from build123d import *

# Parameters (mm, degrees)
SKETCH1_W           = 127
SKETCH1_H           = 101.6
BOSS_EXTRUDE1_DEPTH = 2.54
SKETCH2_W           = 76.2
SKETCH2_H           = 88.9
SKETCH2_W_2         = 34.29
SKETCH2_H_2         = 40.64
BOSS_EXTRUDE2_DEPTH = 6.35
SKETCH3_R           = 2.54
CUT_EXTRUDE1_DEPTH  = 163.763271348
CUT_EXTRUDE2_REACH  = 159.981
SKETCH4_W           = 42.672
SKETCH4_H           = 1.267041817
FILLET1_R           = 3.81
FILLET2_R           = 12.7
SKETCH5_R           = 0.635
CUT_EXTRUDE3_DEPTH  = 163.763271348


with BuildPart() as part:
    # Sketch1 → Boss-Extrude1 (new body)
    with BuildSketch(Plane(origin=(0, 0, 0), x_dir=(1, 0, 0), z_dir=(0, 1, 0))):
        with Locations((63.5, 50.8)):
            Rectangle(SKETCH1_W, SKETCH1_H)
    extrude(amount=BOSS_EXTRUDE1_DEPTH)

    # Sketch2 → Boss-Extrude2 (add)
    with BuildSketch(Plane(origin=(0, 2.54, 0), x_dir=(1, 0, 0), z_dir=(0, 1, 0))):
        with Locations((82.55, 50.8)):
            Rectangle(SKETCH2_W, SKETCH2_H)
        with Locations((64.135, 72.39)):
            Rectangle(SKETCH2_W_2, SKETCH2_H_2, mode=Mode.SUBTRACT)
        with Locations((64.135, 29.21)):
            Rectangle(SKETCH2_W_2, SKETCH2_H_2, mode=Mode.SUBTRACT)
        with Locations((100.965, 29.21)):
            Rectangle(SKETCH2_W_2, SKETCH2_H_2, mode=Mode.SUBTRACT)
        with Locations((100.965, 72.39)):
            Rectangle(SKETCH2_W_2, SKETCH2_H_2, mode=Mode.SUBTRACT)
    extrude(amount=BOSS_EXTRUDE2_DEPTH)

    # Sketch3 → Cut-Extrude1 (cut, through all)
    with BuildSketch(Plane(origin=(0, 2.54, 0), x_dir=(1, 0, 0), z_dir=(0, 1, 0))):
        with Locations(Location((64.135, 72.39, 0), (0, 0, 270))):
            Circle(SKETCH3_R)
        with Locations(Location((100.965, 72.39, 0), (0, 0, 270))):
            Circle(SKETCH3_R)
        with Locations(Location((64.135, 29.21, 0), (0, 0, 270))):
            Circle(SKETCH3_R)
        with Locations(Location((100.965, 29.21, 0), (0, 0, 270))):
            Circle(SKETCH3_R)
    extrude(amount=-CUT_EXTRUDE1_DEPTH, mode=Mode.SUBTRACT)

    # Cut-Extrude2: up to this face of the body (flat: up to its plane)
    cut_extrude2_end = Plane(part.part.faces().sort_by_distance((46.99, 5.715, -29.21))[0])
    # Sketch4 → Cut-Extrude2 (cut, up to the picked face)
    with BuildSketch(Plane(origin=(120.65, 0, 0), x_dir=(0, 0, -1), z_dir=(1, 0, 0)), mode=Mode.PRIVATE) as cut_extrude2_sk1:
        with Locations((72.644, 6.348520909)):
            Rectangle(SKETCH4_W, SKETCH4_H)
    cut_extrude2_tool1 = split(extrude(cut_extrude2_sk1.sketch, amount=-CUT_EXTRUDE2_REACH, mode=Mode.PRIVATE), bisect_by=cut_extrude2_end, keep=Keep.BOTH, mode=Mode.PRIVATE)
    # Sketch4 → Cut-Extrude2 (cut, up to the picked face)
    with BuildSketch(Plane(origin=(120.65, 0, 0), x_dir=(0, 0, -1), z_dir=(1, 0, 0)), mode=Mode.PRIVATE) as cut_extrude2_sk2:
        with Locations((28.956, 6.348520909)):
            Rectangle(SKETCH4_W, SKETCH4_H)
    cut_extrude2_tool2 = split(extrude(cut_extrude2_sk2.sketch, amount=-CUT_EXTRUDE2_REACH, mode=Mode.PRIVATE), bisect_by=cut_extrude2_end, keep=Keep.BOTH, mode=Mode.PRIVATE)
    add(cut_extrude2_tool1.solids().sort_by(Axis((120.65, 6.348521, -72.644), (-1, 0, 0)))[0], mode=Mode.SUBTRACT)
    add(cut_extrude2_tool2.solids().sort_by(Axis((120.65, 6.348521, -28.956), (-1, 0, 0)))[0], mode=Mode.SUBTRACT)

    # Fillet1
    # the kernel refuses this fillet: 3.81 mm, written as the material it takes off along each edge
    with BuildSketch(Plane(origin=(120.65, 2.54, -95.25), x_dir=(0, 0, 1), z_dir=(0, 1, 0)), Plane(origin=(120.65, 2.54, -6.35), x_dir=(-1, 0, 0), z_dir=(0, 1, 0)), Plane(origin=(44.45, 2.54, -6.35), x_dir=(0, 0, -1), z_dir=(0, 1, 0))) as fillet1_piece_1:
        with BuildLine():
            CenterArc((FILLET1_R, -FILLET1_R), FILLET1_R, 90, 90)
            Line((0, -FILLET1_R), (0, 0))
            Line((0, 0), (FILLET1_R, 0))
        make_face()
    extrude(amount=15.875, mode=Mode.SUBTRACT)
    with BuildSketch(Plane(origin=(44.45, 2.54, -95.25), x_dir=(0, 0, 1), z_dir=(0, 1, 0))) as fillet1_piece_2:
        with BuildLine():
            CenterArc((FILLET1_R, FILLET1_R), FILLET1_R, 180, 90)
            Line((0, FILLET1_R), (0, 0))
            Line((0, 0), (FILLET1_R, 0))
        make_face()
    extrude(amount=15.875, mode=Mode.SUBTRACT)

    # Fillet2
    fillet2_edges = [part.edges().sort_by_distance(p)[0] for p in [
        (0, 1.27, -101.6),
        (127, 1.27, -101.6),
        (127, 1.27, 0),
        (0, 1.27, 0),
    ]]
    fillet(fillet2_edges, radius=FILLET2_R)

    # Sketch5 → Cut-Extrude3 (cut, through all)
    with BuildSketch(Plane(origin=(0, 2.54, 0), x_dir=(1, 0, 0), z_dir=(0, 1, 0))):
        with Locations(Location((4.963162708, 5.024067494, 0), (0, 0, 270))):
            Circle(SKETCH5_R)
        with Locations(Location((122.036837292, 5.024067494, 0), (0, 0, 90))):
            Circle(SKETCH5_R)
        with Locations(Location((122.036837292, 96.575932506, 0), (0, 0, 270))):
            Circle(SKETCH5_R)
        with Locations(Location((4.963162708, 96.575932506, 0), (0, 0, 90))):
            Circle(SKETCH5_R)
    extrude(amount=-CUT_EXTRUDE3_DEPTH, mode=Mode.SUBTRACT)


solid = part.part
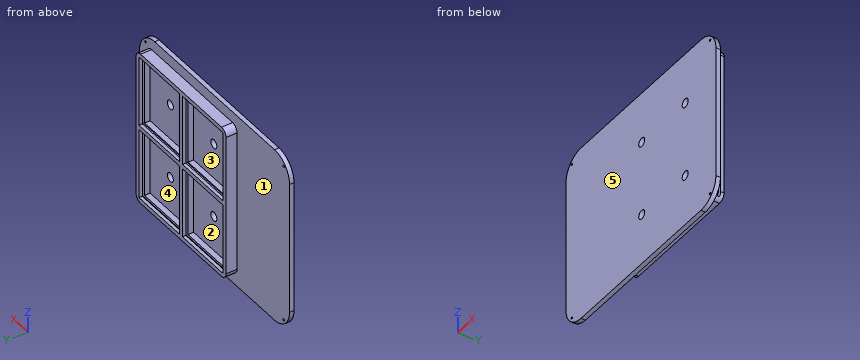
Source: CAD feature listing. Evaluate the final solid. Frame: model axes, mm. Face numbers are marked on the shaded views. A direction names the side the tool comes from. Give positions to 0.01 mm unless a question says otherwise; leave off trailing zeros. Write each loop counter-clockwise with the first axis right and the second up, starting at its lowest first coordinate (ties: lowest second). Pieces come first, ordered by that corner, then holes. Notation, with made-up numbers: M -14,78 L 42,78 A30 ccw 42,116 Z; hole C 67,-38.75 d10. An arc over 180 degrees is marked long. Return JSON: item names as keys, results as strings. Group by question number.
1) Pin query (flat end, axial travel): P1, Ø1.6, axis at x = 56.5, y = 3.5, coming from the +Z side; P2, Ø1.5, axis at x = 59, y = 8.5, coming from the -Z side; P3, Ø1.6, axis at y = 3.5, z = -33, coming from the +X side; P4, Ø3.5, axis at y = 4, z = -26, coming from the -X side. Return the tip coordinate at first contact, or that it passes through.
2) Set-up query: the marked faces 4 and 5. Return all of +Z, -Z, +X, -X, +Y, -Y with unobstructed straight access to the full face (end or side cutting, diameter ignored); none if empty.
3) Cut plane A-A, the plane z = -72.39. Give the number of separate pieces and of enclosed holes in the cut face, plus the area to 3 significant figures.
4) Material intervals for line 1 along Z through (x, y) = (59, 3.25); line 2 along X through (y, z) = (8.75, -71); line 3 along Z through (x, y) = (106, 6.5), sorted ascending. Write a range as [from, to].
5) Pull-direction query (Z, two-part tool) for the marked faces 1, 2 and 3; classes: pulls with the +Z half, pulls with the -Z half, needs draft (parallel to the pull), parting line crosses it, or undercut.
6) Cut plane C-C, the plane x = 26. Output: boundary loops of the cut face in (y, z).
7) Cut plane B-B, the plane z = -59. Output: boundary loops of the cut face in (x, y) (3 decimals).
Recorded:
{
 "1": {"P1": "stops at z = -6.35", "P2": "stops at z = -95.25", "P3": "stops at x = 120.65", "P4": "stops at x = 0"},
 "2": {"face 4": "+Y", "face 5": "+Z, -Z, +X, -X, -Y"},
 "3": {"separate pieces": "5", "enclosed holes": "0", "area": "339 mm²"},
 "4": {"line 1": "z = [-95.25, -92.71], [-52.07, -49.53], [-8.89, -6.35]", "line 2": "x = [44.45, 46.99], [81.28, 83.82], [118.11, 120.65]", "line 3": "z = [-95.25, -93.98], [-51.31, -50.29], [-7.62, -6.35]"},
 "5": {"face 1": "needs draft", "face 2": "undercut", "face 3": "undercut"},
 "6": {"outline": "M 0,-101.6 L 2.54,-101.6 L 2.54,0 L 0,0 Z"},
 "7": {"outline": "M 0,0 L 127,0 L 127,2.54 L 120.65,2.54 L 120.65,5.715 L 118.11,5.715 L 118.11,2.54 L 83.82,2.54 L 83.82,5.715 L 81.28,5.715 L 81.28,2.54 L 46.99,2.54 L 46.99,8.89 L 44.45,8.89 L 44.45,2.54 L 0,2.54 Z; M 81.28,6.982 L 83.82,6.982 L 83.82,8.89 L 81.28,8.89 Z; M 118.11,6.982 L 120.65,6.982 L 120.65,8.89 L 118.11,8.89 Z"}
}
